from build123d import *

# Parameters (mm, degrees)
BOSS_EXTRUDE2_DEPTH = 1.5
SKETCH2_RX          = 2.512468905
SKETCH2_RY          = 2.5
CUT_EXTRUDE1_DEPTH  = 82.304057571


with BuildPart() as part:
    # Sketch1 → Boss-Extrude2 (new body)
    with BuildSketch(Plane(origin=(0, 7.782968327, -77.829683267), x_dir=(1, 0, 0), z_dir=(0, -0.09950371902099842, 0.9950371902099893))):
        with BuildLine():
            Line((-22.056639236, -7.811403035), (-8.5, -7.811403035))
            Line((-8.5, -7.811403035), (-8.5, 72.486835274))
            Line((-8.5, 72.486835274), (-23.140108221, 72.486835274))
            add(Edge.make_bspline(
                [(-23.140108221, 72.486835274), (-33.185752444, 71.376302341), (-35.93451502, 61.602554427)],
                knots=[3.25115225, 3.25115225, 3.25115225, 4.436931985, 4.436931985, 4.436931985], degree=2, weights=[1, 0.829329402, 1]))
            add(Edge.make_bspline(
                [(-35.93451502, 61.602554427), (-36.5, 59.591865073), (-36.5, 57.502405173)],
                knots=[1.295339331, 1.295339331, 1.295339331, 1.570796327, 1.570796327, 1.570796327], degree=2, weights=[1, 0.990530414, 1]))
            Line((-36.5, 57.502405173), (-36.5, 7.253027067))
            add(Edge.make_bspline(
                [(-36.5, 7.253027067), (-36.5, -7.272375759), (-22.056639236, -7.811403035)],
                knots=[4.71238898, 4.71238898, 4.71238898, 6.246067502, 6.246067502, 6.246067502], degree=2, weights=[1, 0.720107382, 1]))
        make_face()
    extrude(amount=BOSS_EXTRUDE2_DEPTH)

    # Sketch2 → Cut-Extrude1 (cut, through all)
    with BuildSketch(Plane(origin=(0, 7.782968327, -77.829683267), x_dir=(-1, 0, 0), z_dir=(0, 0.0995037190209984, -0.9950371902099893))):
        with Locations(Location((18.25, 17.194242647), (0, 0, 90))):
            Ellipse(SKETCH2_RX, SKETCH2_RY)
        with Locations(Location((18.25, 49.856338415), (0, 0, 90))):
            Ellipse(SKETCH2_RX, SKETCH2_RY)
    extrude(amount=-CUT_EXTRUDE1_DEPTH, mode=Mode.SUBTRACT)


solid = part.part
Could you check a few things on this model? Use its own coordinates, in mm. Round coordinates to 2 decimals unless told otherwise and drop trailing zeros. Order: outer loops, then holes, each group sorted by start corner. A loop starts at its lowest first (then second) coordinate and runs counter-clockwise, first axis right, second up.
(1) I'm going to push flat-ended pins straight in: pin 1 (5 mm diameter, centred on y = 23, z = -71.5, fed in from -X); pin 2 (8 mm diameter, centred on x = -22.5, y = 66.5, fed in from -Z); pin 3 (5 mm diameter, centred on x = -21, y = 33.5, fed in from +Z); pin 4 (4 mm diameter, centred on x = -24, y = 13, fed in from +Z). Where does each tip first touch, or does it pass through?
Response values:
pin 1: passes through
pin 2: stops at z = -72.36
pin 3: stops at z = -73.5
pin 4: stops at z = -75.6
(2) Please list where these lines run through material, in increasing order: line 1 along X through (y, z) = (58.5, -71.5); line 2 along Z through (x, y) = (-25, 32.5); line 3 along Z through (x, y) = (-30.25, 41.5).
Response values:
line 1: x = -36.5 to -20.42, -16.08 to -8.5
line 2: z = -75.36 to -73.85
line 3: z = -74.46 to -72.95
(3) Imagine slicing it at A-A (x = -13.25). Write out the boundary of the cut face in (y, z).
Response values:
outline: (-0.14, -77.11) - (0.01, -78.61) - (79.91, -70.62) - (79.76, -69.12) - close
(4) Imagine slicing it at B-B (y = 46). Write out the boundary of the cut face in (x, z), plus the area to 3 significant figures.
Response values:
outline: (-36.5, -74.01) - (-8.5, -74.01) - (-8.5, -72.5) - (-36.5, -72.5) - close
area: 42.2 mm2
